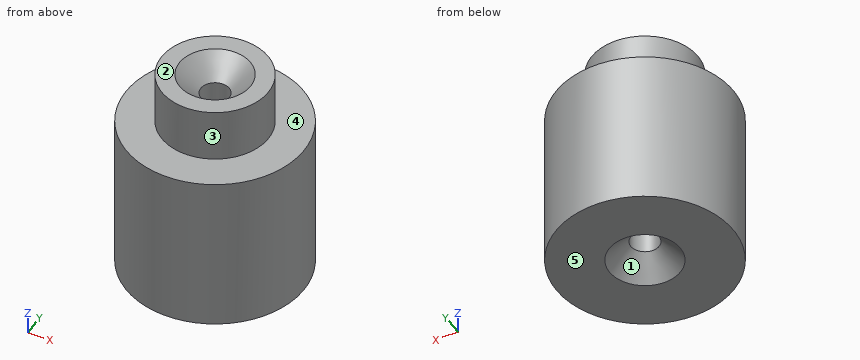
Autodesk Inventor part; units mm, degrees
ref_plane "YZ Plane" through (0, 0, 0) normal (1, 0, 0) x (0, 1, 0)
ref_plane "XZ Plane" through (0, 0, 0) normal (0, 1, 0) x (-1, 0, 0)
ref_plane "XY Plane" through (0, 0, 0) normal (0, 0, 1) x (1, 0, 0)
sketch "Skizze1" plane through (0, 0, 0) normal (0, 0, 1) x (1, 0, 0)
  circle A0 centre (0, 0) radius 5
  dimension "d0" = 10
extrude "Extrusion1" add sketch "Skizze1" against normal blind 9
sketch "Skizze2" plane through (0, 0, 0) normal (0, 0, 1) x (1, 0, 0)
  circle A0 centre (0, 0) radius 3
  dimension "d3" = 6
extrude "Extrusion2" add sketch "Skizze2" along normal blind 3
sketch "Skizze3" plane through (0, 0, 3) normal (0, 0, 1) x (1, 0, 0)
  circle A0 centre (0, 0) radius 3
hole "Bohrung1" at (0, 0, 3) direction (0, 0, -1) diameter 1.6 depth 6 countersink diameter 4 countersink angle 90
sketch "Skizze4" plane through (0, 0, -9) normal (0, 0, -1) x (-1, 0, 0)
  circle A0 centre (0, 0) radius 5
hole "Bohrung2" at (0, 0, -9) direction (0, 0, 1) diameter 1.6 depth 6 countersink diameter 4 countersink angle 90
properties part number "Führungsbüchse" material "Kupfer"
Here's how the part is built. I have some questions about the finished solid (model axes, mm). Face numbers are marked on the shaded views. A direction names the side the tool comes from. Round coordinates to 2 decimals unless told otherwise and drop trailing zeros. Order: outer loops, then holes, each group sorted by start corner. A loop starts at its lowest first (then second) coordinate and runs counter-clockwise, first axis right, second up. Notation, with made-up numbers: (79.25, -39.5) -> (93.25, -39.5) arc R30 ccw to (93.25, -5.5) -> close; hole circle Ø11 at (29, 81.5). An arc over 180 degrees is marked (long way). Use a Markdown table: item, result. Add a question column.
(1) Suppose I cut it at D-D, the plane y = 4.25. Please give me the cut outline in (x, z).
(2) For the marked faces 4 and 5, which set-ups out of +Z, -Z, +X, -X, +Y, -Y let a thin tool reach every point of the face, with its end or its side?
(3) If we mould it in two halves opening along Y, with no side actions, what happens to the marked faces 1, 2 and 3? For each: released by +Y, released by -Y, zero draft, split by the parting line, or undercut.
(4) I need wall thicknesses on line 1 along Y through (x, z) = (0, -5.7); line 2 along Y through (x, z) = (0, 0.8); line 3 along Z through (x, y) = (-4, 1.5). Which ranges of each line are inside material? Lowest first, please.
(5) For pin 1 Ø1 at (y, z) = (-4, -2) entering from -X; pin 2 Ø3 at (y, z) = (-2, 1) entering from +X; pin 3 Ø6 at (x, z) = (-0.5, -0.5) entering from +Y; pin 4 Ø2 at (x, y) = (0, 0) entering from -Z, each with a flat end and sliding along its axis, tell me the tip position at first contact or that it passes through.
(6) Suppose I cut it at A-A, the plane x = 0. Please give me the cut outline in (y, z), and give its area (3 significant figures).
(7) Suppose I cut it at C-C, the plane y = -2.25. Please give me the cut outline in (x, z).
Verdict:
| question | item | result |
|---|---|---|
| 1 | outline | (-2.63, -9) -> (2.63, -9) -> (2.63, 0) -> (-2.63, 0) -> close |
| 2 | face 4 | +Z |
| 2 | face 5 | -Z, +X, -X, +Y, -Y |
| 3 | face 1 | undercut |
| 3 | face 2 | zero draft |
| 3 | face 3 | split by the parting line |
| 4 | line 1 | -5 to -0.8, 0.8 to 5 |
| 4 | line 2 | -3 to -0.8, 0.8 to 3 |
| 4 | line 3 | -9 to 0 |
| 5 | pin 1 | x = -3.57 |
| 5 | pin 2 | x = 4.92 |
| 5 | pin 3 | y = 5 |
| 5 | pin 4 | z = -8 |
| 6 | outline | (-5, -9) -> (-2, -9) -> (-0.8, -7.8) -> (-0.8, 1.8) -> (-2, 3) -> (-3, 3) -> (-3, 0) -> (-5, 0) -> close; (0.8, -7.8) -> (2, -9) -> (5, -9) -> (5, 0) -> (3, 0) -> (3, 3) -> (2, 3) -> (0.8, 1.8) -> close |
| 6 | area | 85.9 mm2 |
| 7 | outline | (-4.47, -9) -> (4.47, -9) -> (4.47, 0) -> (1.98, 0) -> (1.98, 3) -> (-1.98, 3) -> (-1.98, 0) -> (-4.47, 0) -> close |
